from build123d import *

# Parameters (mm, degrees)
F0_R     = 24.106038
F0_R_2   = 10.411348
F0_R_3   = 13.98419
F1_DEPTH = 25


with BuildPart() as f1:
    # F0 (on Front) → F1 (new body)
    with BuildSketch(Plane.XZ):
        with BuildLine():
            Line((4.137931, 24.655172), (0, 25))
            ThreePointArc((0, 25), (-25, 0), (0, -25))
            Line((0, -25), (4.105443, -24.660603))
            ThreePointArc((4.105443, -24.660603), (19.074015, -16.161125), (25, 0))
            ThreePointArc((25, 0), (19.084657, 16.148556), (4.137931, 24.655172))
        make_face()
        Circle(F0_R, mode=Mode.SUBTRACT)
        with BuildLine():
            ThreePointArc((4.137931, 24.655172), (2.076137, 24.913644), (0, 25))
            Line((0, 25), (4.137931, 24.655172))
        make_face()
        with BuildLine():
            Line((4.105443, -24.660603), (0, -25))
            ThreePointArc((0, -25), (2.059724, -24.915006), (4.105443, -24.660603))
        make_face()
        with BuildLine():
            Line((90, 17.5), (4.137931, 24.655172))
            ThreePointArc((4.137931, 24.655172), (19.084657, 16.148556), (25, 0))
            ThreePointArc((25, 0), (19.074015, -16.161125), (4.105443, -24.660603))
            Line((4.105443, -24.660603), (91.441807, -17.440504))
            ThreePointArc((91.441807, -17.440504), (72.51488, -0.721517), (90, 17.5))
        make_face()
        with BuildLine():
            ThreePointArc((107.5, 0), (102.374369, 12.374369), (90, 17.5))
            ThreePointArc((90, 17.5), (72.51488, -0.721517), (91.441807, -17.440504))
            ThreePointArc((91.441807, -17.440504), (102.874036, -11.853657), (107.5, 0))
        make_face()
        with Locations((90, 0)):
            Circle(F0_R_2, mode=Mode.SUBTRACT)
        Circle(F0_R)
        Circle(F0_R_3, mode=Mode.SUBTRACT)
    extrude(amount=F1_DEPTH)


solid = f1.part
Verification items for the finished model (mm, model axes). Coordinates: 2 decimals unless noted, no trailing zeros. Order: outer loops, then holes, each group sorted by start corner. A loop starts at its lowest first (then second) coordinate and runs counter-clockwise, first axis right, second up. Notation, with made-up numbers: (10.25, -34) -> (56.25, -34) arc R37 cw to (56.25, 4) -> close; hole circle Ø3 at (80.5, 54.5). An arc over 180 degrees is marked (long way). Put each result on its own line as item: value. Start each with the question number.
1. Cross-section at B-B, the plane z = 5.5. Record the boundary of the cut face in (x, y), then the cut area to 3 significant figures.
2. Material ranges on L1, parallel to X at y = -6.5, z = 1.5; L2, parallel to X at y = -18.75, z = -8; L3, parallel to Z at x = 81, y = -12.5, recorded low to high. Write a range as [from, to].
3. Go/stop test with flat-tipped pins: pin 1 Ø10 at (y, z) = (-5, 8.5) entering from +X; pin 2 Ø2 at (x, y) = (25.5, -12.5) entering from +Z; pin 3 Ø8 at (x, z) = (37, -9) entering from +Y; pin 4 Ø3 at (x, y) = (-8.5, -21) entering from +Z. Record where each tip stops, or that it passes through.
4. Cross-section at C-C, the plane x = 77. Record the boundary of the cut face in (y, z).
5. Cross-section at A-A, the plane y = -17. Record the boundary of the cut face in (x, z).
6. Cross-section at D-D, the plane z = 22. Record the boundary of the cut face in (x, y), then the cut area to 3 significant figures.
7. Mould release check, pull along X, two halves, no side actions. Record for faces 1 (the cylindrical face through (2.031, -12.325, -24.917)), 2 (the flat face through (40, -25, 0)), 3 (the cylindrical face through (7.52, -12.32, 11.79)), 4 (the cylindrical face through (99.617, -12.325, -3.988)): released by +X, released by -X, zero draft, split by the parting line, or undercut.
Computed:
1. outline: (-24.39, -25) -> (-12.86, -25) -> (-12.86, 0) -> (-24.39, 0) -> close; (12.86, -25) -> (81.16, -25) -> (81.16, 0) -> (12.86, 0) -> close; (98.84, -25) -> (106.61, -25) -> (106.61, 0) -> (98.84, 0) -> close
1. area: 2,190 mm2
2. L1: [-24.95, -13.9], [13.9, 79.7], [100.3, 107.44]
2. L2: [-23.69, -11.47], [11.47, 83.34], [96.66, 105.56]
2. L3: [-18.3, -5.23], [5.23, 18.25]
3. pin 1: x = 107.15
3. pin 2: z = 22.96
3. pin 3: y = 0
3. pin 4: z = 24
4. outline: (-25, -18.63) -> (0, -18.63) -> (0, 18.58) -> (-25, 18.58) -> close
5. outline: (0, -25) arc R25 ccw to (4.11, -24.66) -> (91.44, -17.44) arc R17.5 ccw to (107.5, 0) arc R17.5 ccw to (90, 17.5) -> (4.14, 24.66) arc R25 ccw to (0, 25) arc R25 ccw to start; hole circle Ø27.97 at (0, 0); hole circle Ø20.82 at (90, 0)
6. outline: (-11.87, -25) -> (36, -25) -> (36, 0) -> (-11.87, 0) -> close
6. area: 1,200 mm2
7. face 1: released by +X
7. face 2: zero draft
7. face 3: undercut
7. face 4: undercut
